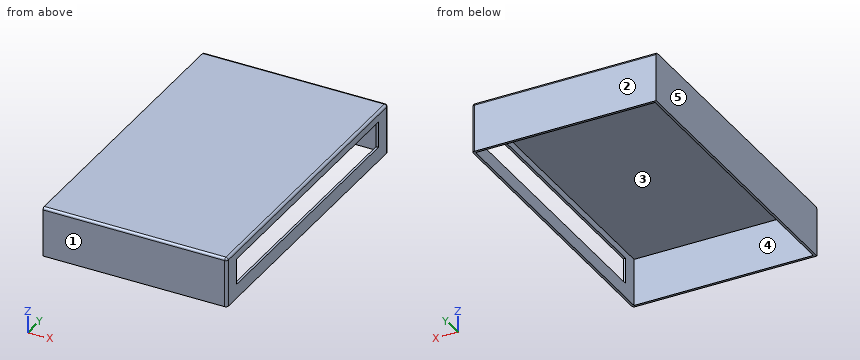
Autodesk Inventor part; units mm, degrees
ref_plane "YZ Plane" through (0, 0, 0) normal (1, 0, 0) x (0, 1, 0)
ref_plane "XZ Plane" through (0, 0, 0) normal (0, 1, 0) x (-1, 0, 0)
ref_plane "XY Plane" through (0, 0, 0) normal (0, 0, 1) x (1, 0, 0)
sketch "Skizze1" plane through (0, 0, 0) normal (0, 0, 1) x (1, 0, 0)
  line L0 (-38.75, -63) -> (38.75, -63)
  line L1 (38.75, -63) -> (38.75, 63)
  line L2 (38.75, 63) -> (-38.75, 63)
  line L3 (-38.75, 63) -> (-38.75, -63)
  line L4 (-38.75, -63) -> (38.75, 63) construction
  line L5 (38.75, -63) -> (-38.75, 63) construction
  point P0 (0, 0)
  dimension "d23" = 77.5
  dimension "d24" = 126
extrude "Grundkörper" add sketch "Skizze1" along normal blind 21
sketch "Skizze6" plane through (0, 0, 0) normal (0, 0, -1) x (-1, 0, 0)
  line L0 (-37.75, -62) -> (37.75, -62)
  line L1 (37.75, -62) -> (37.75, 62)
  line L2 (37.75, 62) -> (-37.75, 62)
  line L3 (-37.75, 62) -> (-37.75, -62)
  line L4 (-37.75, -62) -> (37.75, 62) construction
  line L5 (37.75, -62) -> (-37.75, 62) construction
  line L6 (-38.75, 63) -> (38.75, 63)
  line L7 (38.75, 63) -> (38.75, -63)
  point P0 (0, 0)
  dimension "d27" = 1
  dimension "d28" = 1
extrude "Ausschnitt" cut sketch "Skizze6" against normal blind 20
sketch "Skizze8" plane through (38.75, -63, 0) normal (1, 0, 0) x (0, 0, -1)
  line L0 (0, 0) -> (-21, 0) construction
  line L1 (0, 0) -> (0, 126) construction
  line L2 (0, 126) -> (-21, 126) construction
  line L3 (-21, 0) -> (-21, 126) construction
  line L4 (-25.2, 63) -> (4.2, 63) construction
  line L5 (-6, 7.5) -> (-17, 7.5)
  line L6 (-17, 7.5) -> (-17, 118.5)
  line L7 (-17, 118.5) -> (-6, 118.5)
  line L8 (-6, 118.5) -> (-6, 7.5)
  line L9 (-6, 7.5) -> (-17, 118.5) construction
  line L10 (-17, 7.5) -> (-6, 118.5) construction
  point P0 (0, 63)
  point P1 (-11.5, 63)
  dimension "d32" = 7.5
  dimension "d33" = 6
  dimension "d34" = 4
extrude "Anschlüsse" cut sketch "Skizze8" against normal up to surface (1 mm away)
fillet "Rundung2" radius 1 5 edges at (38.75, 0, 21) (0, 63, 21) (0, -63, 21) (38.75, -63, 10.5) (38.75, 63, 10.5)
equation "\"d28\" = d27"
properties part number "800-20-MOTOR-CONTROLLER-BLD-300B-02" material "Aluminium 6061"
Model file for the job. Use its own axes, mm. Face numbers are marked on the shaded views. A direction names the side the tool comes from. Coordinates: 2 decimals unless noted, no trailing zeros. Loops run counter-clockwise (first coordinate to the right, second up) from the corner with the lowest first, then second, coordinate; pieces in that order, holes last. Notation, with made-up numbers: (21.5, 69.25) - (46.5, 69.25) arc R7 ccw to (46.5, 75.25) - close; hole circle Ø5 at (38, 75). An arc over 180 degrees is marked (long way). Write item = value, one per line. Start each with the question number.
Item 1: Wall check: probe 1 along Y at (x, z) = (-35, 19.25); probe 2 along X at (y, z) = (51.5, 5.5); probe 3 along Z at (x, y) = (-9, 55.5). Give the ranges that are in metal, low to high. Write a range as [from, to].
Item 2: Drop flat-ended pins along their axis: pin 1 Ø22.5 at (x, y) = (10, -28.5) entering from -Z; pin 2 Ø1.1 at (x, z) = (38.5, 9.5) entering from -Y; pin 3 Ø8 at (y, z) = (11.5, 12) entering from +X. Give the stop position or say it passes through.
Item 3: 3-axis set-ups, long thin cutter, end or side, ignore diameter. For the marked faces 4 and 5: which of +Z, -Z, +X, -X, +Y, -Y reach the whole face in a straight line?
Item 4: Pull direction Y, two halves, no side cores. Call the marked faces 1, 2 and 3: +Y half, -Y half, draft (parallel to the pull), parting line (faces both ways), or undercut.
Item 5: Saw through at A-A, the plane z = 3.5. List the corners of the cut face in (x, y), then the cut area to 3 significant figures.
Item 6: Saw through at B-B, the plane y = 20. List the corners of the cut face in (x, z).
Item 7: Saw through at D-D, the plane x = 9.5. List the corners of the cut face in (y, z).
Item 8: Saw through at C-C, the plane z = 13. List the corners of the cut face in (x, y), then the cut area to 3 significant figures.
Answers:
q1.probe_1 = [-63, -62], [62, 63]
q1.probe_2 = [-38.75, -37.75], [37.75, 38.75]
q1.probe_3 = [20, 21]
q2.pin_1 = 20
q2.pin_2 = -62.98
q2.pin_3 = -37.75
q3.face_4 = -Z
q3.face_5 = +Z, -Z, -X, +Y, -Y
q4.face_1 = -Y half
q4.face_2 = +Y half
q4.face_3 = undercut
q5.outline = (-38.75, -63) - (37.75, -63) arc R1 ccw to (38.75, -62) - (38.75, 62) arc R1 ccw to (37.75, 63) - (-38.75, 63) - close; hole (-37.75, -62) - (37.75, -62) - (37.75, 62) - (-37.75, 62) - close
q5.area = 403 mm2
q6.outline = (-38.75, 0) - (-37.75, 0) - (-37.75, 20) - (37.75, 20) - (37.75, 17) - (38.75, 17) - (38.75, 20) arc R1 ccw to (37.75, 21) - (-38.75, 21) - close; (37.75, 0) - (38.75, 0) - (38.75, 6) - (37.75, 6) - close
q7.outline = (-63, 0) - (-62, 0) - (-62, 20) - (62, 20) - (62, 0) - (63, 0) - (63, 20) arc R1 ccw to (62, 21) - (-62, 21) arc R1 ccw to (-63, 20) - close
q8.outline = (-38.75, -63) - (37.75, -63) arc R1 ccw to (38.75, -62) - (38.75, -55.5) - (37.75, -55.5) - (37.75, -62) - (-37.75, -62) - (-37.75, 62) - (37.75, 62) - (37.75, 55.5) - (38.75, 55.5) - (38.75, 62) arc R1 ccw to (37.75, 63) - (-38.75, 63) - close
q8.area = 292 mm2
